For this review, take the finished solid that the model builds, in its own axes (mm). A direction names the side the tool comes from. Coordinates: 2 decimals unless noted, no trailing zeros. Loops run counter-clockwise (first coordinate to the right, second up) from the corner with the lowest first, then second, coordinate; pieces in that order, holes last. Notation, with made-up numbers: M -2,87.25 L 13,87.25 A16 cw 13,107.25 Z; hole C -9,78.5 d6. An arc over 180 degrees is marked long. Put each result on its own line as item: value.
```python
from build123d import *

# Parameters (mm, degrees)
SKETCH1_R           = 1.5
BOSS_EXTRUDE1_DEPTH = 6


with BuildPart() as part:
    # Sketch1 → Boss-Extrude1 (new body)
    with BuildSketch(Plane.XY):
        with BuildLine():
            Line((8.319591794, -4), (0.599591794, -4))
            ThreePointArc((0.599591794, -4), (-1.930230334, -3.098386677), (-3.319591794, -0.8))
            Line((-3.319591794, -0.8), (-3.319591794, 3.2))
            Line((-3.319591794, 3.2), (-1.800408206, 3.2))
            ThreePointArc((-1.800408206, 3.2), (1.004202752, 3.979483631), (3.594535859, 2.651473185))
            Line((3.594535859, 2.651473185), (3.594535859, -1.348526815))
            Line((3.594535859, -1.348526815), (8.319591794, -1.348526815))
            Line((8.319591794, -1.348526815), (8.319591794, -4))
        make_face()
        with Locations((0.599591794, 0)):
            Circle(SKETCH1_R, mode=Mode.SUBTRACT)
    extrude(amount=BOSS_EXTRUDE1_DEPTH)


solid = part.part
```
(1) Add section D-D (x = 5.5). Write out the cut boundary in (y, z), plus the area to 3 significant figures.
Determined:
outline: M -4,0 L -1.35,0 L -1.35,6 L -4,6 Z
area: 15.9 mm^2
(2) Wall thickness on line 1 along Y through (x, z) = (3, 1); line 2 along Y through (x, z) = (0.5, 1.15); line 3 along Y through (x, z) = (4, 1.8): over which ranges is each line inside the solid? List them lowest first. Write a range as [from, to].
Determined:
line 1: y = [-4, 3.2]
line 2: y = [-4, -1.5], [1.5, 4]
line 3: y = [-4, -1.35]
(3) Draft analysis for pull direction Y (two halves, no side actions). For faces 1 (the cylindrical face through (-1.9, -3.122, 2.958)), 2 (the flat face through (-3.32, 1, 3)), 3 (the cylindrical face through (2.03, 0.45, 2.96)), 4 (the cylindrical face through (0.963, 3.983, 2.958)), state which applies: +Y half, -Y half, draft (parallel to the pull), parting line (faces both ways), or undercut.
Determined:
face 1: -Y half
face 2: draft
face 3: undercut
face 4: +Y half
(4) Tool access review of faces 5 (the flat face through (-3, 3.2, 3)), 6 (the flat face through (3.595, 1, 3)), 7 (the flat face through (3, -1, 0)): name each direction out of +Z, -Z, +X, -X, +Y, -Y from which nothing blocks a thin tool from reaching the whole face with its end or side.
Determined:
face 5: +Z, -Z, -X, +Y
face 6: +Z, -Z, +X, +Y
face 7: -Z, +X, -X, +Y, -Y
(5) Add section B-B (z = 5.2). Write out the cut boundary in (x, y).
Determined:
outline: M -3.32,-0.8 A4 ccw 0.6,-4 L 8.32,-4 L 8.32,-1.35 L 3.59,-1.35 L 3.59,2.65 A4 ccw -1.8,3.2 L -3.32,3.2 Z; hole C 0.6,0 d3
(6) Add section A-A (y = 0). Write out the cut boundary in (x, z), plus the area to 3 significant figures.
Determined:
outline: M -3.32,0 L -0.9,0 L -0.9,6 L -3.32,6 Z; M 2.1,0 L 3.59,0 L 3.59,6 L 2.1,6 Z
area: 23.5 mm^2
(7) For pin 1 (1.7 mm diameter, centred on x = -2.5, z = 3.5, fed in from +Y); pin 2 (2.5 mm diameter, centred on x = 6, z = 4.5, fed in from +Y); pin 3 (3 mm diameter, centred on y = 0.5, z = 3.5, fed in from +X), all flat-tipped, find the tip position at first contact; note any pin that passes through.
Determined:
pin 1: stops at y = 3.31
pin 2: stops at y = -1.35
pin 3: stops at x = 3.59
(8) Add section C-C (x = 1.5). Write out the cut boundary in (y, z).
Determined:
outline: M -4,0 L -1.2,0 L -1.2,6 L -4,6 Z; M 1.2,0 L 3.9,0 L 3.9,6 L 1.2,6 Z
